```python
from build123d import *

# Parameters (mm, degrees)
CROQUIS1_R                   = 115
SALIENTE_EXTRUIR1_DEPTH      = 140
SALIENTE_EXTRUIR2_DEPTH      = 80
SALIENTE_EXTRUIR2_DEPTH_BACK = 80
CROQUIS2_R                   = 290
CROQUIS2_R_2                 = 115
REDONDEO1_R                  = 30
REDONDEO2_R                  = 5
REDONDEO3_R                  = 5


with BuildPart() as part:
    # Croquis1 → Saliente-Extruir1 (new body)
    with BuildSketch(Plane(origin=(0, 0, 0), x_dir=(1, 0, 0), z_dir=(0, 1, 0))):
        with Locations(Location((0, 0, 0), (0, 0, 270))):
            Circle(CROQUIS1_R)
    extrude(amount=SALIENTE_EXTRUIR1_DEPTH)

    # Croquis2 → Saliente-Extruir2 (add, two sides: drawn at the far end of the back side and taken through both)
    with BuildSketch(Plane(origin=(0, 70, 0), x_dir=(1, 0, 0), z_dir=(0, 1, 0)).offset(-SALIENTE_EXTRUIR2_DEPTH_BACK)):
        with Locations(Location((0, 0, 0), (0, 0, 270))):
            Circle(CROQUIS2_R)
        with Locations(Location((0, 0, 0), (0, 0, 270))):
            Circle(CROQUIS2_R_2, mode=Mode.SUBTRACT)
    extrude(amount=SALIENTE_EXTRUIR2_DEPTH + SALIENTE_EXTRUIR2_DEPTH_BACK)

    # Redondeo1
    redondeo1_edges = [part.edges().sort_by_distance(p)[0] for p in [
        (0, -10, -290),
        (0, 150, -290),
    ]]
    fillet(redondeo1_edges, radius=REDONDEO1_R)

    # Redondeo2
    redondeo2_edges = [part.edges().sort_by_distance(p)[0] for p in [
        (0, -10, -115),
    ]]
    fillet(redondeo2_edges, radius=REDONDEO2_R)

    # Redondeo3
    redondeo3_edges = [part.edges().sort_by_distance(p)[0] for p in [
        (0, 150, -115),
    ]]
    fillet(redondeo3_edges, radius=REDONDEO3_R)


solid = part.part
```
Model file for the job. Use its own axes, mm. A direction names the side the tool comes from. Give positions to 0.01 mm unless a question says otherwise; leave off trailing zeros. Loops run counter-clockwise (first coordinate to the right, second up) from the corner with the lowest first, then second, coordinate; pieces in that order, holes last. Notation, with made-up numbers: (-21, 29.25) -> (12, 29.25) arc R26 ccw to (12, 51.25) -> close; hole circle Ø7 at (-17.75, -19). An arc over 180 degrees is marked (long way). Write each question's results on one line, items separated by ' | '.
(1) Cut at B-B on z = 0. List the corners of the cut face in (x, y), and give its area (3 significant figures).
Geometry results:
outline: (-290, 20) arc R30 ccw to (-260, -10) -> (-120, -10) arc R5 ccw to (-115, -5) -> (-115, 0) -> (115, 0) -> (115, -5) arc R5 ccw to (120, -10) -> (260, -10) arc R30 ccw to (290, 20) -> (290, 120) arc R30 ccw to (260, 150) -> (120, 150) arc R5 ccw to (115, 145) -> (115, 140) -> (-115, 140) -> (-115, 145) arc R5 ccw to (-120, 150) -> (-260, 150) arc R30 ccw to (-290, 120) -> close | area: 87,400 mm²
(2) Flat gauge pins, fed straight in: pin 1 Ø12 at (y, z) = (16, 92.5) entering from +X; pin 2 Ø2 at (y, z) = (130, -150) entering from -X; pin 3 Ø1 at (y, z) = (125, 24) entering from +X. Where does each tip first touch, or does it go through?
Geometry results:
pin 1: stops at x = 276.63 | pin 2: stops at x = -246.91 | pin 3: stops at x = 288.68
(3) Probe line 1 along X through (y, z) = (144, 0); line 2 along X through (y, z) = (141.55, 0); line 3 along X through (y, z) = (69, 4). List the from-to ranges inside material, lowest first.
Geometry results:
line 1: x = -278 to -115, 115 to 278 | line 2: x = -280.87 to -115, 115 to 280.87 | line 3: x = -289.97 to 289.97
(4) Tool access for faces 1 (the flat face through (2, 0, -2)), 2 (the flat face through (-54, -10, 112)), 3 (the flat face through (2, 140, -2)): list every direction of +Z, -Z, +X, -X, +Y, -Y with a clear straight run to the whole face (end or side of a thin tool).
Geometry results:
face 1: -Y | face 2: +Z, -Z, +X, -X, -Y | face 3: +Y
(5) Cut at A-A on x = 0. List the corners of the cut face in (y, z).
Geometry results:
outline: (-10, -260) arc R30 ccw to (20, -290) -> (120, -290) arc R30 ccw to (150, -260) -> (150, -120) arc R5 ccw to (145, -115) -> (140, -115) -> (140, 115) -> (145, 115) arc R5 ccw to (150, 120) -> (150, 260) arc R30 ccw to (120, 290) -> (20, 290) arc R30 ccw to (-10, 260) -> (-10, 120) arc R5 ccw to (-5, 115) -> (0, 115) -> (0, -115) -> (-5, -115) arc R5 ccw to (-10, -120) -> close
(6) Pull direction Z, two halves, no side cores. Call faces 4 (the cylindrical face through (87.108, 69.3, 276.608)), 5 (the cylindrical face through (-112.265, 142.465, -24.93)), 6 (the flat face through (-54, 150, 112)): released by +Z, released by -Z, zero draft, split by the parting line, or undercut.
Geometry results:
face 4: split by the parting line | face 5: undercut | face 6: zero draft
(7) Cut at C-C on y = 110. List the corners of the cut face in (x, z).
Geometry results:
outline: circle Ø580 at (0, 0)
